from build123d import *

# Parameters (mm, degrees)
F0_W           = 5
F0_H           = 260
F1_DEPTH       = 28
F0_W_2         = 95
F2_DEPTH       = 23
F3_D           = 8.5
F4_D           = 6.8
F5_D           = 11
F5_CBORE_D     = 19
F5_CBORE_DEPTH = 13


# Not quite as in the source:
# - a feature names something its author has since deleted; it is built from what else it names


with BuildPart() as f1:
    # F0 (on Front) → F1 (new body)
    with BuildSketch(Plane.XZ):
        with Locations((-47.5, 0)):
            Rectangle(F0_W, F0_H)
    extrude(amount=F1_DEPTH)

    # F0 (on Front) → F2 (join)
    with BuildSketch(Plane.XZ):
        with Locations((2.5, 0)):
            Rectangle(F0_W_2, F0_H)
    extrude(amount=F2_DEPTH)

    # F3 (through all)
    with Locations(Plane(origin=(0, 0, 0), x_dir=(1, 0, 0), z_dir=(0, 1, 0))):
        with Locations((41, -90), (-41, -90), (41, -35), (-41, -35)):
            Hole(F3_D / 2)

    # F4 (through all)
    with Locations(Plane(origin=(0, 0, 0), x_dir=(1, 0, 0), z_dir=(0, 1, 0))):
        with Locations((19, 5), (-19, 5), (19, 45), (-19, 45), (19, 115), (-19, 115)):
            Hole(F4_D / 2)

    # F5 (through all)
    with Locations(Plane(origin=(0, 0, 0), x_dir=(1, 0, 0), z_dir=(0, 1, 0))):
        with Locations((36, -109), (-36, -109), (36, -57), (-36, -57), (36, 57), (-36, 57), (-36, 109), (36, 109)):
            CounterBoreHole(F5_D / 2, F5_CBORE_D / 2, F5_CBORE_DEPTH)


solid = f1.part
Model file for the job. Use its own axes, mm. A direction names the side the tool comes from. Round coordinates to 2 decimals unless told otherwise and drop trailing zeros. Order: outer loops, then holes, each group sorted by start corner. A loop starts at its lowest first (then second) coordinate and runs counter-clockwise, first axis right, second up. Notation, with made-up numbers: M 16.5,20.25 L 59.5,20.25 A24 cw 59.5,48.25 Z; hole C -4.5,-18 d4. An arc over 180 degrees is marked long. Write each question's results on one line, items separated by ' | '. Start each with the question number.
(1) Saw through at A-A, the plane z = 57. Give the cut face in (x, y).
(2) Two-plate mould, pull along Z, no slides. Class faces 4 (the face through (-32, -13, -53)), 5 (the face through (-1, -11, -130)), 6 (the face through (-48, -28, 2)): pulls with the +Z half, pulls with the -Z half, needs draft (parallel to the pull), parting line crosses it, or undercut.
(3) Saw through at B-B, the plane y = -10. State how many separate pieces and enclosed holes the cut face has, then the cut area to 3 significant figures.
(4) Saw through at D-D, the plane x = -11.5. Give the cut face in (y, z), then the cut area to 3 significant figures.
(5) Drop flat-ended pins along their axis: pin 1 (15 mm diameter, centred on x = 38.5, z = 54.5, fed in from +Y); pin 2 (17 mm diameter, centred on x = -36, z = -57, fed in from -Y); pin 3 (17.5 mm diameter, centred on x = -36, z = 109, fed in from +Y). Give the stop position or say it passes through.
(6) Saw through at C-C, the plane x = 19. Give the cut face in (y, z), then the cut area to 3 significant figures.
(7) Probe probe 1 along X at (y, z) = (-16, 109); probe 2 along Z at (x, y) = (19, -9.5); probe 3 along X at (y, z) = (-6.75, -6). List the from-to ranges inside material, lowest first. Write a range as from..to.
(8) Which spindle directions (+Z, -Z, +X, -X, +Y, -Y) get a long thin tool onto all of the face, cutting with end or side? Do faces 1 (the face through (40, -13, 113)), 2 (the face through (-45, -25, 62)), 3 (the face through (-16.494, -11.661, -7.298)). Say none if no direction does.
Established:
1) outline: M -50,-28 L -45,-28 L -45,-23 L -41.5,-23 L -41.5,-13 L -45.5,-13 L -45.5,0 L -50,0 Z; M -30.5,-23 L 30.5,-23 L 30.5,-13 L 26.5,-13 L 26.5,0 L -26.5,0 L -26.5,-13 L -30.5,-13 Z; M 41.5,-23 L 50,-23 L 50,0 L 45.5,0 L 45.5,-13 L 41.5,-13 Z
2) face 4: undercut | face 5: pulls with the -Z half | face 6: needs draft
3) separate pieces: 1 | enclosed holes: 18 | area: 23,300 mm^2
4) outline: M -23,-130 L 0,-130 L 0,130 L -23,130 Z | area: 5,980 mm^2
5) pin 1: stops at y = 0 | pin 2: stops at y = -23 | pin 3: stops at y = -13
6) outline: M -23,-130 L 0,-130 L 0,-118.4 L -23,-118.4 Z; M -23,-111.6 L 0,-111.6 L 0,-48.4 L -23,-48.4 Z; M -23,-41.6 L 0,-41.6 L 0,-8.4 L -23,-8.4 Z; M -23,-1.6 L 0,-1.6 L 0,130 L -23,130 Z | area: 5,510 mm^2
7) probe 1: x = -50..-41.5, -30.5..30.5, 41.5..50 | probe 2: z = -130..-118.4, -111.6..-48.4, -41.6..-8.4, -1.6..130 | probe 3: x = -50..-22.25, -15.75..15.75, 22.25..50
8) face 1: +Y | face 2: +Z, -Z, +X, -Y | face 3: +Y, -Y
